Source: CAD feature listing. Evaluate the final solid. Frame: model axes, mm. Face numbers are marked on the shaded views. A direction names the side the tool comes from. Coordinates: 2 decimals unless noted, no trailing zeros. Order: outer loops, then holes, each group sorted by start corner. A loop starts at its lowest first (then second) coordinate and runs counter-clockwise, first axis right, second up.
Autodesk Inventor part; units mm, degrees
ref_plane "Work Plane1" through (3.5, 0, 0) normal (0, 0, 1) x (1, 0, 0)
ref_plane "YZ Plane" through (0, 0, 0) normal (1, 0, 0) x (0, 1, 0)
ref_plane "XZ Plane" through (0, 0, 0) normal (0, 1, 0) x (-1, 0, 0)
sketch "Sketch1" plane through (0, 0, 0) normal (0, 0, 1) x (1, 0, 0)
  line L0 (0, 9.906) -> (0, 4.7625)
  line L1 (19.05, 4.7625) -> (127, 4.7625)
  line L2 (127, 4.7625) -> (127, 0)
  line L3 (127, 0) -> (-1.6002, 0)
  line L4 (0, -1.9812) -> (0, 11.8872)
  line L5 (-27.3202, 0) -> (152.72, 0)
  line L6 (-1.6002, 0) -> (-1.6002, 9.906)
  line L7 (-1.6002, 9.906) -> (0, 9.906)
  line L8 (19.05, 4.7625) -> (18.2562, 4.7625)
  line L9 (18.2562, 4.7625) -> (0, 4.7625)
  dimension "d0" = 127
  dimension "d1" = 107.95
  dimension "d2" = 9.525
  dimension "d8" = 1.6002
  dimension "d9" = 19.812
  dimension "d15" = 9.525
  dimension "d16" = 0.7937
revolve "Body" add sketch "Sketch1" angle 360 about axis through (127, 0, 0) along (-1, 0, 0)
sketch "Sketch2" plane through (0, 0, 0) normal (1, 0, 0) x (0, 0, -1)
  circle A0 centre (0, 0) radius 9.906
  line L0 (0, 8.2416) -> (7.1374, 4.1208)
  line L1 (7.1374, 4.1208) -> (7.1374, -4.1208)
  line L2 (7.1374, -4.1208) -> (0, -8.2416)
  line L3 (0, -8.2416) -> (-7.1374, -4.1208)
  line L4 (-7.1374, -4.1208) -> (-7.1374, 4.1208)
  line L5 (-7.1374, 4.1208) -> (0, 8.2416)
  circle A1 centre (0, 0) radius 9.906
  dimension "d10" = 14.2748
extrude "Head" add sketch "Sketch2" against normal blind 7.493 contours L0 L1 L2 L3 L4 L5
sketch "Sketch3" plane through (0, 0, 0) normal (0, 0, 1) x (1, 0, 0)
  line L0 (-7.493, 7.1374) -> (-7.493, 8.2416)
  line L1 (-7.493, 8.2416) -> (-6.8555, 8.2416)
  line L2 (-6.8555, 8.2416) -> (-7.493, 7.1374)
  line L3 (-2.8347, 8.2416) -> (-7.493, 8.2416)
  line L4 (-7.493, 8.2416) -> (-7.493, 5.9322)
  line L5 (-1.6002, 8.2416) -> (-7.493, 8.2416)
  line L6 (-7.493, 8.2416) -> (-7.493, 4.1208)
  line L7 (-8.6716, 0) -> (-0.4216, 0)
  dimension "d5" = 30
  dimension "d18" = 14.2748
revolve "Chamfer1" cut sketch "Sketch3" angle 360 about axis through (-10, 0, 0) along (1, 0, 0)
thread "Thread"
chamfer "Chamfer2" distance 0.7938 distance2 0.7938 1 edges at (127, -4.7625, 0) measured on face at (127, -1.1883, 1.0527)
ref_plane "Work Plane1" through (3.5, 0, 0) normal (0, 0, 1) x (1, 0, 0)
equation "\"d0\" = NLG"
equation "\"d1\" = GEL"
equation "\"d2\" = GD"
equation "\"d8\" = PHH"
equation "\"d9\" = LADI"
equation "\"d15\" = BDM"
equation "\"d16\" = GAL"
equation "\"d10\" = SW"
equation "\"d3\" = KOH"
equation "\"d13\" = GEL"
equation "\"d6\" = -0.5 * SPD + 0.5 * GD"
equation "\"d7\" = -0.5 * SPD + 0.5 * GD"
equation "\"d5\" = ANG1"
equation "\"d18\" = SW0"
equation "\"NLG\" = 127"
equation "\"GD\" = NND"
equation "\"BDM\" = NND"
equation "\"KOH\" = 7.493"
equation "\"GEL\" = 107.95"
equation "\"LADI\" = 19.812"
equation "\"SW\" = 14.2748"
equation "\"PHH\" = 1.6002"
equation "\"SW0\" = 14.2748"
equation "\"SPD\" = GD1"
equation "\"ANG1\" = 30deg"
equation "\"GAL\" = 0.79375"
equation "\"GUL\" = GAL"
equation "\"GD1\" = 7.9375"
equation "\"THREADDIA\" = 9.525"
equation "\"SDH\" = SW"
equation "\"TOA\" = 30deg"
equation "\"RR\" = 0.09525"
equation "\"NND\" = 9.525"
equation "\"SD\" = 0"
equation "\"SD2\" = NND"
equation "\"E0\" = 16.48739"
properties part number "ANSI B18.6.3 - 3/8-16 UNC x 5, PHWHMSI" material "Steel, Mild"
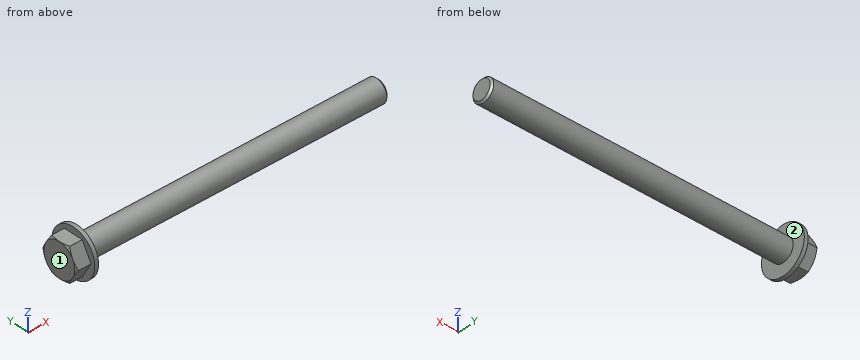
1. Section query A-A, the plane x = 27. Output: boundary loops of the cut face in (y, z) (1 decimal), plus the area to 3 significant figures.
2. Material intervals for line 1 along X through (y, z) = (1.25, -8.75); line 2 along X through (y, z) = (5, -4.5); line 3 along Y through (x, z) = (62.5, -0.5), sorted ascending.
3. Access query for the marked faces 1 and 2. Directions: +Z, -Z, +X, -X, +Y, -Y. A direction counts if a zero-diameter tool reaches every point of the face in a straight line with its end or side. Return the directions, or none.
4. Contact query for flat-ended pins moving along their axis: P1, Ø5, axis at x = 94, y = -1.5, coming from the -Z side; P2, Ø8, axis at x = 6, z = 2.5, coming from the -Y side; P3, Ø6, axis at y = 3, z = 4, coming from the +X side; P4, Ø6.5, axis at x = -6, y = -0.5, coming from the -Z side. Output: stop coordinate, or through.
Answer key:
1. outline: circle Ø9.5 at (0, 0)
1. area: 71.3 mm2
2. line 1: x = -1.6 to 0
2. line 2: x = -7.49 to 0
2. line 3: y = -4.74 to 4.74
3. face 1: +Z, -Z, -X, +Y, -Y
3. face 2: +X
4. P1: stops at z = -4.76
4. P2: stops at y = -4.76
4. P3: stops at x = 127
4. P4: stops at z = -7.14
